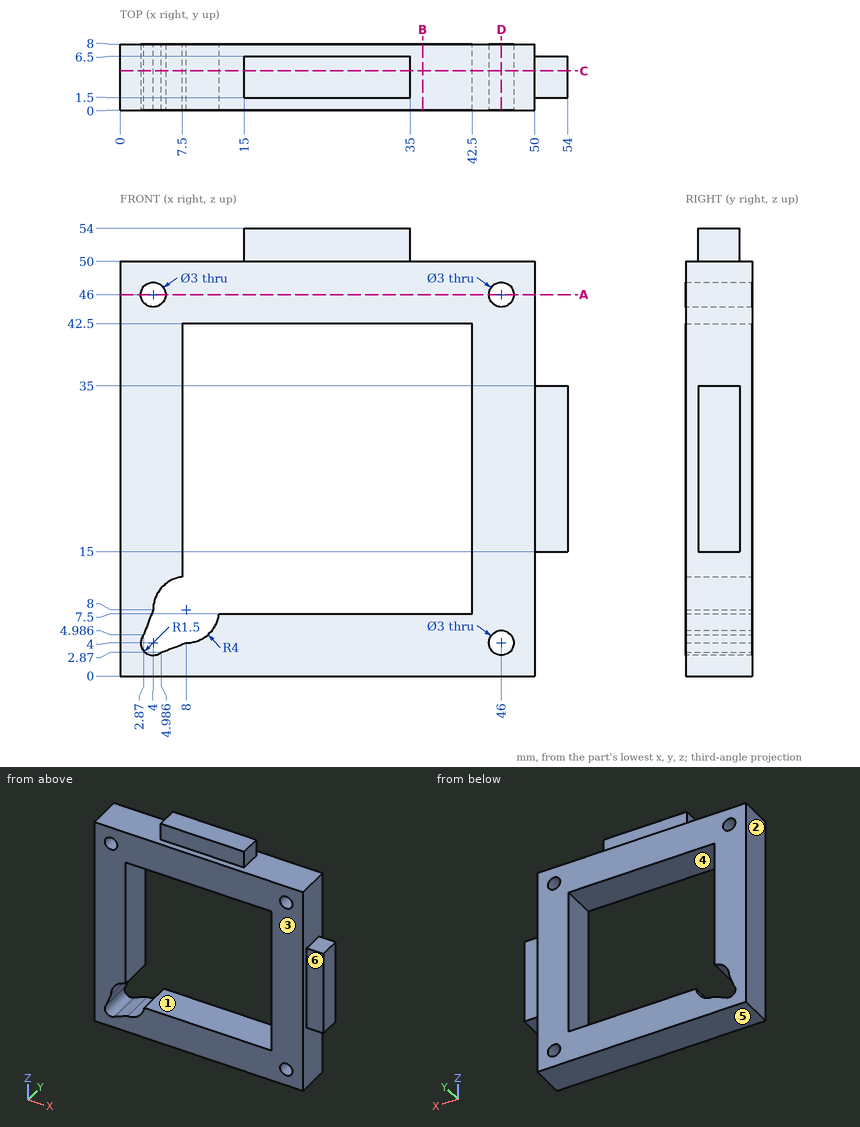
Source: three-view drawing plus pictorial views. Frame: mm from the lowest corner of the part. A direction names the side the tool comes from. Coordinates: 2 decimals unless noted, no trailing zeros. Order: outer loops, then holes, each group sorted by start corner. A loop starts at its lowest first (then second) coordinate and runs counter-clockwise, first axis right, second up. Notation, with made-up numbers: M 39.5,11.5 L 92.5,11.5 A18 cw 92.5,36.5 Z; hole C 77.25,26.5 d1. An arc over 180 degrees is marked long. One line per question, with ' | ' between items.
Item 1: Draft query along X for the marked faces 1, 2 and 3. Return one class per face: released by +X, released by -X, zero draft, split by the parting line, or undercut.
Geometry results:
face 1: undercut | face 2: released by -X | face 3: zero draft
Item 2: Section A-A (z = 46). Output: boundary loops of the cut face in (x, y), then the cut area to 3 significant figures.
Geometry results:
outline: M 0,0 L 2.5,0 L 2.5,8 L 0,8 Z; M 5.5,0 L 44.5,0 L 44.5,8 L 5.5,8 Z; M 47.5,0 L 50,0 L 50,8 L 47.5,8 Z | area: 352 mm^2
Item 3: Section C-C (y = 4.75). Output: boundary loops of the cut face in (x, z).
Geometry results:
outline: M 0,0 L 50,0 L 50,15 L 54,15 L 54,35 L 50,35 L 50,50 L 35,50 L 35,54 L 15,54 L 15,50 L 0,50 Z; hole C 4,46 d3; hole M 2.87,4.99 A1.5 ccw 4.99,2.87 L 8,4 A4 ccw 11.97,7.5 L 42.5,7.5 L 42.5,42.5 L 7.5,42.5 L 7.5,11.97 A4 ccw 4,8 Z; hole C 46,4 d3; hole C 46,46 d3
Item 4: Reachability of the marked faces 4, 5 and 6 from +Z, -Z, +X, -X, +Y, -Y: full face, straight path, thin tool, end or side. Return the list, or none.
Geometry results:
face 4: +Y, -Y | face 5: -Z, +X, -X, +Y, -Y | face 6: +Z, -Z, +X, -Y
Item 5: Ray query, line 1 along X through (y, z) = (3.25, 46); line 2 along X through (y, z) = (3, 27); line 3 along Z through (x, y) = (27.5, 6.75). Return the intervals inside material, ascending.
Geometry results:
line 1: x = 0 to 2.5, 5.5 to 44.5, 47.5 to 50 | line 2: x = 0 to 7.5, 42.5 to 54 | line 3: z = 0 to 7.5, 42.5 to 50
Item 6: Section D-D (x = 46). Output: boundary loops of the cut face in (y, z).
Geometry results:
outline: M 0,0 L 8,0 L 8,2.5 L 0,2.5 Z; M 0,5.5 L 8,5.5 L 8,44.5 L 0,44.5 Z; M 0,47.5 L 8,47.5 L 8,50 L 0,50 Z
Item 7: Pin query (flat end, axial travel): pin 1 (3 mm diameter, centred on x = 52, y = 3, fed in from +Z); pin 2 (3 mm diameter, centred on x = 52, z = 22.5, fed in from +Y); pin 3 (3 mm diameter, centred on y = 2, z = 12, fed in from +X); pin 4 (2 mm diameter, centred on x = 41, z = 31, fed in from -Y). Return the tip coordinate at first contact, or that it passes through.
Geometry results:
pin 1: stops at z = 35 | pin 2: stops at y = 6.5 | pin 3: stops at x = 50 | pin 4: passes through
Item 8: Section B-B (x = 36.5). Output: boundary loops of the cut face in (y, z), then the cut area to 3 significant figures.
Geometry results:
outline: M 0,0 L 8,0 L 8,7.5 L 0,7.5 Z; M 0,42.5 L 8,42.5 L 8,50 L 0,50 Z | area: 120 mm^2
